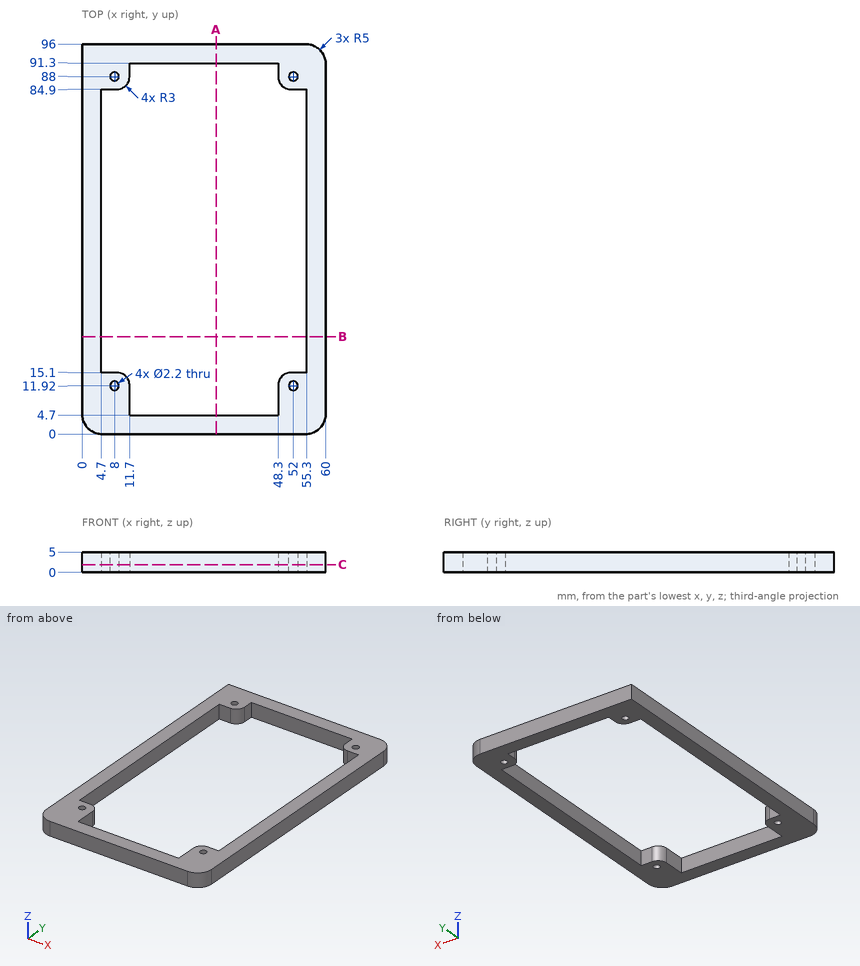
Print and shaded views of the part. All mm, measured from the part's lowest x, y and z. Round coordinates to 2 decimals unless told otherwise and drop trailing zeros. Order: outer loops, then holes, each group sorted by start corner. A loop starts at its lowest first (then second) coordinate and runs counter-clockwise, first axis right, second up.
Q1. Slice it at B-B (y = 24). Write the cut outline in (x, z).
Q2. Slice it at C-C (z = 1.9). Write the cut outline in (x, y), and give its area (3 significant figures).
Q3. Drop a flat-ended pin along its axis: pin 1 (2 mm diameter, centred on x = 8, y = 88, fed in from -Z). Give the stop position or say it passes through.
Q4. Wall check: L1, parallel to Y at x = 52, z = 1.85; L2, parallel to Y at x = 6.5, z = 4; L3, parallel to Y at x = 39.5, z = 4.8. Give the ranges that are in metal, low to high.
Q5. Slice it at A-A (x = 33). Write the cut outline in (y, z), and give its area (3 significant figures).
Results below:
1. outline: (0, 0) - (4.7, 0) - (4.7, 5) - (0, 5) - close; (55.3, 0) - (60, 0) - (60, 5) - (55.3, 5) - close
2. outline: (0, 5) arc R5 ccw to (5, 0) - (55, 0) arc R5 ccw to (60, 5) - (60, 91) arc R5 ccw to (55, 96) - (0, 96) - close; hole (4.7, 15.1) - (8.7, 15.1) arc R3 cw to (11.7, 12.1) - (11.7, 4.7) - (48.3, 4.7) - (48.3, 12.1) arc R3 cw to (51.3, 15.1) - (55.3, 15.1) - (55.3, 84.9) - (51.3, 84.9) arc R3 cw to (48.3, 87.9) - (48.3, 91.3) - (11.7, 91.3) - (11.7, 87.9) arc R3 cw to (8.7, 84.9) - (4.7, 84.9) - close; hole circle Ø2.2 at (8, 11.92); hole circle Ø2.2 at (8, 88); hole circle Ø2.2 at (52, 11.92); hole circle Ø2.2 at (52, 88)
2. area: 1,570 mm2
3. pin 1: passes through
4. L1: y = 0 to 10.82, 13.02 to 15.1, 84.9 to 86.9, 89.1 to 96
4. L2: y = 0 to 15.1, 84.9 to 96
4. L3: y = 0 to 4.7, 91.3 to 96
5. outline: (0, 0) - (4.7, 0) - (4.7, 5) - (0, 5) - close; (91.3, 0) - (96, 0) - (96, 5) - (91.3, 5) - close
5. area: 47.0 mm2
